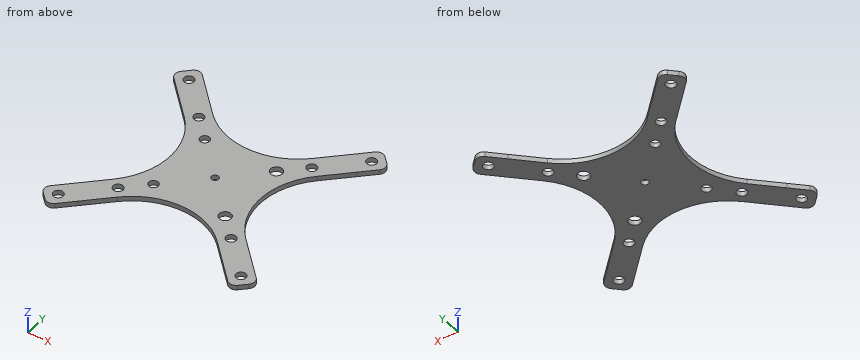
```python
from build123d import *

# Parameters (mm, degrees)
CROQUIS1_R              = 2
CROQUIS1_R_2            = 2.1
CROQUIS1_R_3            = 2.5
CROQUIS1_R_4            = 1.5
SALIENTE_EXTRUIR1_DEPTH = 2
REDONDEO3_R             = 3


with BuildPart() as part:
    # Croquis1 → Saliente-Extruir1 (new body)
    with BuildSketch(Plane.XY):
        with BuildLine():
            Line((-31.096194078, 38.16726189), (-21.213203436, 28.284271247))
            ThreePointArc((-21.213203436, 28.284271247), (0, 19.497474683), (21.213203436, 28.284271247))
            Line((21.213203436, 28.284271247), (31.096194078, 38.16726189))
            Line((31.096194078, 38.16726189), (38.890872965, 45.961940777))
            Line((38.890872965, 45.961940777), (42.426406871, 42.426406871))
            Line((42.426406871, 42.426406871), (45.961940777, 38.890872965))
            Line((45.961940777, 38.890872965), (38.16726189, 31.096194078))
            Line((38.16726189, 31.096194078), (28.284271247, 21.213203436))
            ThreePointArc((28.284271247, 21.213203436), (19.497474683, 0), (28.284271247, -21.213203436))
            Line((28.284271247, -21.213203436), (38.16726189, -31.096194078))
            Line((38.16726189, -31.096194078), (45.961940777, -38.890872965))
            Line((45.961940777, -38.890872965), (42.426406871, -42.426406871))
            Line((42.426406871, -42.426406871), (38.890872965, -45.961940777))
            Line((38.890872965, -45.961940777), (31.096194078, -38.16726189))
            Line((31.096194078, -38.16726189), (21.213203436, -28.284271247))
            ThreePointArc((21.213203436, -28.284271247), (0, -19.497474683), (-21.213203436, -28.284271247))
            Line((-21.213203436, -28.284271247), (-31.096194078, -38.16726189))
            Line((-31.096194078, -38.16726189), (-38.890872965, -45.961940777))
            Line((-38.890872965, -45.961940777), (-42.426406871, -42.426406871))
            Line((-42.426406871, -42.426406871), (-45.961940777, -38.890872965))
            Line((-45.961940777, -38.890872965), (-38.16726189, -31.096194078))
            Line((-38.16726189, -31.096194078), (-28.284271247, -21.213203436))
            ThreePointArc((-28.284271247, -21.213203436), (-19.497474683, 0), (-28.284271247, 21.213203436))
            Line((-28.284271247, 21.213203436), (-38.16726189, 31.096194078))
            Line((-38.16726189, 31.096194078), (-45.961940777, 38.890872965))
            Line((-45.961940777, 38.890872965), (-42.426406871, 42.426406871))
            Line((-42.426406871, 42.426406871), (-38.890872965, 45.961940777))
            Line((-38.890872965, 45.961940777), (-31.096194078, 38.16726189))
        make_face()
        with Locations((-15.25, 15.25)):
            Circle(CROQUIS1_R, mode=Mode.SUBTRACT)
        with Locations((-24.04163056, 24.04163056)):
            Circle(CROQUIS1_R_2, mode=Mode.SUBTRACT)
        with Locations((-38.890872965, 38.890872965)):
            Circle(CROQUIS1_R_2, mode=Mode.SUBTRACT)
        with Locations(Location((38.890872965, 38.890872965, 0), (0, 0, 180))):
            Circle(CROQUIS1_R_2, mode=Mode.SUBTRACT)
        with Locations(Location((24.04163056, 24.04163056, 0), (0, 0, 180))):
            Circle(CROQUIS1_R_2, mode=Mode.SUBTRACT)
        with Locations(Location((15.25, 15.25, 0), (0, 0, 180))):
            Circle(CROQUIS1_R_3, mode=Mode.SUBTRACT)
        with Locations((15.25, -15.25)):
            Circle(CROQUIS1_R_3, mode=Mode.SUBTRACT)
        with Locations((24.04163056, -24.04163056)):
            Circle(CROQUIS1_R_2, mode=Mode.SUBTRACT)
        with Locations((38.890872965, -38.890872965)):
            Circle(CROQUIS1_R_2, mode=Mode.SUBTRACT)
        with Locations(Location((-15.25, -15.25, 0), (0, 0, 180))):
            Circle(CROQUIS1_R, mode=Mode.SUBTRACT)
        with Locations(Location((-24.04163056, -24.04163056, 0), (0, 0, 180))):
            Circle(CROQUIS1_R_2, mode=Mode.SUBTRACT)
        with Locations(Location((-38.890872965, -38.890872965, 0), (0, 0, 180))):
            Circle(CROQUIS1_R_2, mode=Mode.SUBTRACT)
        Circle(CROQUIS1_R_4, mode=Mode.SUBTRACT)
    extrude(amount=SALIENTE_EXTRUIR1_DEPTH)

    # Redondeo3
    redondeo3_edges = [part.edges().sort_by_distance(p)[0] for p in [
        (-38.890872965, 45.961940777, 1),
        (38.890872965, 45.961940777, 1),
        (45.961940777, 38.890872965, 1),
        (45.961940777, -38.890872965, 1),
        (38.890872965, -45.961940777, 1),
        (-38.890872965, -45.961940777, 1),
        (-45.961940777, -38.890872965, 1),
        (-45.961940777, 38.890872965, 1),
    ]]
    fillet(redondeo3_edges, radius=REDONDEO3_R)


solid = part.part
```
Part model, mm, in its own coordinate system. Round coordinates to 2 decimals unless told otherwise and drop trailing zeros. Order: outer loops, then holes, each group sorted by start corner. A loop starts at its lowest first (then second) coordinate and runs counter-clockwise, first axis right, second up. Notation, with made-up numbers: M -33,41.25 L 25,41.25 A35 ccw 25,75.25 Z; hole C 81,-13.5 d2. An arc over 180 degrees is marked long. Put each result on its own line as item: value. Start each with the question number.
1. Drop flat-ended pins along their axis: pin 1 (1 mm diameter, centred on x = -31.5, z = 1.5, fed in from -Y); pin 2 (2.5 mm diameter, centred on x = -15.25, y = -15.25, fed in from +Z); pin 3 (1 mm diameter, centred on y = 23, z = 1.5, fed in from -X). Give the stop position or say it passes through.
2. Slice it at B-B on y = 15.25. List the corners of the cut face in (x, z).
3. Slice it at C-C on x = -35.5. List the corners of the cut face in (y, z).
4. Slice it at D-D on z = 0.3. State how many separate pieces and enclosed holes the cut face has, then the cut area to 3 significant figures.
5. Drill centre lines: probe 1 along X at (y, z) = (-25, 1.4); probe 2 along X at (y, z) = (23, 0.7); probe 3 along X at (y, z) = (-14, 0.55). Where is each one in solid material? Low to high. Write a range as [from, to].
6. Slice it at A-A on x = -15.25. List the corners of the cut face in (y, z).
Findings:
1. pin 1: y = -39.07
1. pin 2: through
1. pin 3: x = -30.57
2. outline: M -23.66,0 L -17.25,0 L -17.25,2 L -23.66,2 Z; M -13.25,0 L 12.75,0 L 12.75,2 L -13.25,2 Z; M 17.75,0 L 23.66,0 L 23.66,2 L 17.75,2 Z
3. outline: M -42.57,0 L -28.43,0 L -28.43,2 L -42.57,2 Z; M 28.43,0 L 42.57,0 L 42.57,2 L 28.43,2 Z
4. separate pieces: 1
4. enclosed holes: 13
4. area: 2,870 mm2
5. probe 1: [-32.07, -25.91], [-22.17, -17.32], [17.32, 22.17], [25.91, 32.07]
5. probe 2: [-30.07, -25.87], [-22.22, -14.07], [14.07, 22.22], [25.87, 30.07]
5. probe 3: [-22.96, -16.81], [-13.69, 13.08], [17.42, 22.96]
6. outline: M -23.66,0 L -17.25,0 L -17.25,2 L -23.66,2 Z; M -13.25,0 L 13.25,0 L 13.25,2 L -13.25,2 Z; M 17.25,0 L 23.66,0 L 23.66,2 L 17.25,2 Z
